from build123d import *

# Parameters (mm, degrees)
ESQUISSE1_W      = 74
ESQUISSE1_H      = 66
ESQUISSE1_R      = 1.5
EXTRUSION1_DEPTH = 2
ESQUISSE2_R      = 1.5
EXTRUSION2_DEPTH = 10


with BuildPart() as part:
    # Esquisse1 → Extrusion1 (new body)
    with BuildSketch(Plane.XY):
        with Locations((8.831885794, -13.706808511)):
            Rectangle(ESQUISSE1_W, ESQUISSE1_H)
        with Locations((-18.168114206, 9.293191489)):
            Circle(ESQUISSE1_R, mode=Mode.SUBTRACT)
        with Locations((-18.168114206, -36.706808511)):
            Circle(ESQUISSE1_R, mode=Mode.SUBTRACT)
        with Locations((38.331885794, -5.206808511)):
            Circle(ESQUISSE1_R, mode=Mode.SUBTRACT)
        with Locations((38.331885794, -27.206808511)):
            Circle(ESQUISSE1_R, mode=Mode.SUBTRACT)
        with Locations((38.331885794, -16.206808511)):
            Circle(ESQUISSE1_R, mode=Mode.SUBTRACT)
    extrude(amount=EXTRUSION1_DEPTH)

    # Esquisse2 → Extrusion2 (cut)
    with BuildSketch(Plane.XY.offset(2)):
        with Locations((27.831885794, -10.706808511)):
            Circle(ESQUISSE2_R)
        with Locations((-4.168114206, -10.706808511)):
            Circle(ESQUISSE2_R)
        with Locations((-4.168114206, -42.706808511)):
            Circle(ESQUISSE2_R)
        with Locations((27.831885794, -42.706808511)):
            Circle(ESQUISSE2_R)
    extrude(amount=-EXTRUSION2_DEPTH, mode=Mode.SUBTRACT)


solid = part.part
The model under review builds one solid part; all positions refer to its coordinate system, in mm. Round coordinates to 2 decimals unless told otherwise and drop trailing zeros. Write item = value, one per line. Start each with the question number.
Item 1: Clearance check with a flat-ended pin moving along its axis: pin 1 Ø5 at (x, y) = (34, 2.5) entering from -Z. State where the tip first meets the part, or that it passes through.
Item 2: Mouldability with a two-part tool opening along X and no side actions: class faces 1 (the face through (8, -13, 0)), 2 (the face through (45.832, -14, 1)), 3 (the face through (-28.168, -14, 1)), 4 (the face through (37.23, -26.19, 0.99)) as released by +X, released by -X, zero draft, split by the parting line, or undercut.
Item 3: For line 1 along X through (y, z) = (-9.5, 1.75); line 2 along X through (y, z) = (8.5, 1.65); line 3 along X through (y, z) = (9.5, 0.35), list the stretches that pass through material, from the lowest coordinate up.
Conclusion:
q1.pin_1 = 0
q2.face_1 = zero draft
q2.face_2 = released by +X
q2.face_3 = released by -X
q2.face_4 = undercut
q3.line_1 = -28.17 to -5.06, -3.28 to 26.94, 28.72 to 45.83
q3.line_2 = -28.17 to -19.44, -16.89 to 45.83
q3.line_3 = -28.17 to -19.65, -16.68 to 45.83
